Here's the drawing with two shaded views (mm, measured from the low corner). I have some questions. Coordinates: 2 decimals unless noted, no trailing zeros. Loops run counter-clockwise (first coordinate to the right, second up) from the corner with the lowest first, then second, coordinate; pieces in that order, holes last. Notation, with made-up numbers: (-34.5, -24) -> (11.5, -24) arc R15 cw to (11.5, -12) -> close; hole circle Ø5 at (2, 83). An arc over 180 degrees is marked (long way). Answer as a JSON object with one key per item and string values. Group by question number.
Q1. Thinking about a two-plate mould opening in X: for the marked faces 1, 2, 3 and 4, which applies, released by +X, released by -X, zero draft, split by the parting line, or undercut?
Q2. I want a section at A-A on y = 9. Write out the boundary of the cut face in (x, z), then the cut area to 3 significant figures.
Q3. I need wall thicknesses on line 1 (X direction, y = 9, z = 0.6); line 2 (Y direction, x = 49, z = 0.65); line 3 (X direction, y = 10.25, z = 2.85). Which ranges of each line are inside material? Lowest first, please.
Q4. I'm going to push flat-ended pins straight in: pin 1 (1.5 mm diameter, centred on x = 51, z = 1.5, fed in from -Y); pin 2 (6 mm diameter, centred on x = 9, y = 9, fed in from -Z); pin 3 (10.5 mm diameter, centred on x = 49, y = 9, fed in from +Z). Where does each tip first touch, or does it pass through?
Q5. I want a section at D-D on y = 6.75. Count the separate pieces of the cut face and the enclosed holes in it, then the cut area to 3 significant figures.
Q6. I want a section at C-C on z = 3.35. Write out the boundary of the cut face in (x, y).
Q7. I want a section at B-B on x = 9. Write out the boundary of the cut face in (y, z).
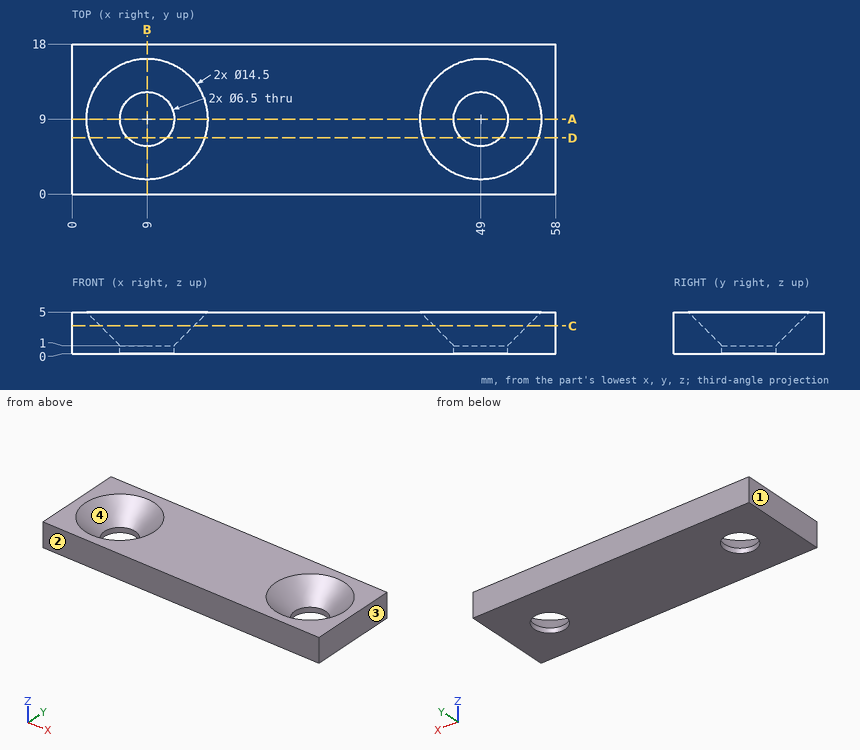
Result set:
{
 "1": {"face 1": "released by -X", "face 2": "zero draft", "face 3": "released by +X", "face 4": "undercut"},
 "2": {"outline": "(0, 0) -> (5.75, 0) -> (5.75, 1) -> (1.75, 5) -> (0, 5) -> close; (12.25, 0) -> (45.75, 0) -> (45.75, 1) -> (41.75, 5) -> (16.25, 5) -> (12.25, 1) -> close; (52.25, 0) -> (58, 0) -> (58, 5) -> (56.25, 5) -> (52.25, 1) -> close", "area": "193 mm²"},
 "3": {"line 1": "x = 0 to 5.75, 12.25 to 45.75, 52.25 to 58", "line 2": "y = 0 to 5.75, 12.25 to 18", "line 3": "x = 0 to 4.06, 13.94 to 44.06, 53.94 to 58"},
 "4": {"pin 1": "stops at y = 0", "pin 2": "passes through", "pin 3": "stops at z = 3"},
 "5": {"separate pieces": "3", "enclosed holes": "0", "area": "205 mm²"},
 "6": {"outline": "(0, 0) -> (58, 0) -> (58, 18) -> (0, 18) -> close; hole circle Ø11.2 at (9, 9); hole circle Ø11.2 at (49, 9)"},
 "7": {"outline": "(0, 0) -> (5.75, 0) -> (5.75, 1) -> (1.75, 5) -> (0, 5) -> close; (12.25, 0) -> (18, 0) -> (18, 5) -> (16.25, 5) -> (12.25, 1) -> close"}
}
